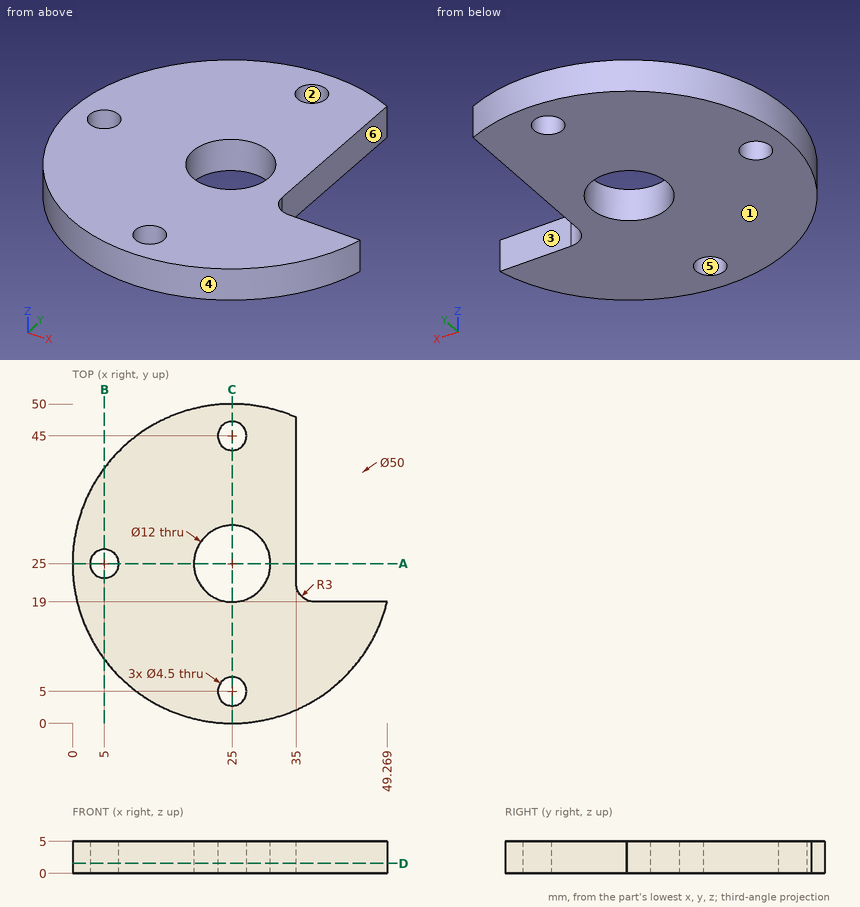
Part print with two shaded views. Sizes in mm from the minimum x, y, z corner. A direction names the side the tool comes from. Round coordinates to 2 decimals unless told otherwise and drop trailing zeros. Order: outer loops, then holes, each group sorted by start corner. A loop starts at its lowest first (then second) coordinate and runs counter-clockwise, first axis right, second up. Notation, with made-up numbers: M -13,32.5 L 4,32.5 A25 cw 4,61.5 Z; hole C 7,-17.75 d5. An arc over 180 degrees is marked long. Put each result on its own line as item: value. Start each with the question number.
1. Slice it at B-B on x = 5. List the corners of the cut face in (y, z), then the cut area to 4 significant figures.
2. Drop flat-ended pins along their axis: pin 1 (7 mm diameter, centred on x = 25, y = 45, fed in from +Z); pin 2 (2.5 mm diameter, centred on y = 30, z = 1.5, fed in from +X); pin 3 (1.5 mm diameter, centred on x = 44, z = 3.5, fed in from +Y); pin 4 (1.5 mm diameter, centred on x = 15.5, z = 1.5, fed in from +Y). Give the stop position or say it passes through.
3. Slice it at A-A on y = 25. List the corners of the cut face in (x, z), then the cut area to 3 significant figures.
4. Slice it at D-D on z = 1.55. List the corners of the cut face in (x, y), then the cut area to 3 significant figures.
5. Slice it at C-C on x = 25. List the corners of the cut face in (y, z).
6. Two-plate mould, pull along Y, no slides. Class the marked faces 1, 2, 3 and 4: +Y half, -Y half, draft (parallel to the pull), parting line (faces both ways), or undercut.
7. Drill centre lines: probe 1 along Y at (x, z) = (25, 1.75); probe 2 along X at (y, z) = (27, 2.45) (1 decimal); probe 3 along X at (y, z) = (24.5, 1.7) (1 decimal). Where is each one in solid material? Low to high. Write a range as [from, to].
8. Tool access for the marked faces 5 and 6: list every direction of +Z, -Z, +X, -X, +Y, -Y with a clear straight run to the whole face (end or side of a thin tool).
Findings:
1. outline: M 10,0 L 22.75,0 L 22.75,5 L 10,5 Z; M 27.25,0 L 40,0 L 40,5 L 27.25,5 Z
1. area: 127.5 mm2
2. pin 1: z = 5
2. pin 2: x = 35
2. pin 3: y = 19
2. pin 4: y = 48.42
3. outline: M 0,0 L 2.75,0 L 2.75,5 L 0,5 Z; M 7.25,0 L 19,0 L 19,5 L 7.25,5 Z; M 31,0 L 35,0 L 35,5 L 31,5 Z
3. area: 92.5 mm2
4. outline: M 35,22 L 35,47.91 A25 ccw long 49.27,19 L 38,19 A3 cw Z; hole C 5,25 d4.5; hole C 25,25 d12; hole C 25,5 d4.5; hole C 25,45 d4.5
4. area: 1,470 mm2
5. outline: M 0,0 L 2.75,0 L 2.75,5 L 0,5 Z; M 7.25,0 L 19,0 L 19,5 L 7.25,5 Z; M 31,0 L 42.75,0 L 42.75,5 L 31,5 Z; M 47.25,0 L 50,0 L 50,5 L 47.25,5 Z
6. face 1: draft
6. face 2: undercut
6. face 3: +Y half
6. face 4: parting line
7. probe 1: [0, 2.75], [7.25, 19], [31, 42.75], [47.25, 50]
7. probe 2: [0.1, 4], [6, 19.3], [30.7, 35]
7. probe 3: [0, 2.8], [7.2, 19], [31, 35]
8. face 5: +Z, -Z
8. face 6: +Z, -Z, +X, +Y
